Input: part model. Units: mm. Frame: model coordinates. Give positions to 0.01 mm unless a question says otherwise; leave off trailing zeros. Loops run counter-clockwise (first coordinate to the right, second up) from the corner with the lowest first, then second, coordinate; pieces in that order, holes last. Notation, with made-up numbers: (22, -37) -> (35, -37) arc R11 cw to (35, -19) -> close; hole circle Ø5 at (-17.5, 66). An arc over 180 degrees is marked (long way). Use CSV: the item, a comma, the result in double quotes.
```python
from build123d import *

# Parameters (mm, degrees)
SKETCH_1_R                       = 40.5
SKETCH_1_R_2                     = 34
SKETCH_1_R_3                     = 1.5
EXTRUDE_1_DEPTH                  = 2
CUT_EXTRUDE_1_DEPTH              = 58.310557492
FILLET_1_R                       = 1
PATTERN_CIRCULAR_1_COUNT         = 11
FILLET_1_OF_PATTERN_CIRCULAR_1_R = 1


with BuildPart() as part:
    # Sketch 1 → Extrude 1 (new body)
    with BuildSketch(Plane.XY):
        Circle(SKETCH_1_R)
        Circle(SKETCH_1_R_2, mode=Mode.SUBTRACT)
        with Locations((0, -38)):
            Circle(SKETCH_1_R_3, mode=Mode.SUBTRACT)
        with Locations((-20.544351063, -31.967634248)):
            Circle(SKETCH_1_R_3, mode=Mode.SUBTRACT)
        with Locations((-34.566015823, -15.785770494)):
            Circle(SKETCH_1_R_3, mode=Mode.SUBTRACT)
        with Locations((-37.613214791, 5.407963854)):
            Circle(SKETCH_1_R_3, mode=Mode.SUBTRACT)
        with Locations((-28.718483825, 24.88470789)):
            Circle(SKETCH_1_R_3, mode=Mode.SUBTRACT)
        with Locations((-10.70583716, 36.460732997)):
            Circle(SKETCH_1_R_3, mode=Mode.SUBTRACT)
        with Locations((10.70583716, 36.460732997)):
            Circle(SKETCH_1_R_3, mode=Mode.SUBTRACT)
        with Locations((28.718483825, 24.88470789)):
            Circle(SKETCH_1_R_3, mode=Mode.SUBTRACT)
        with Locations((37.613214791, 5.407963854)):
            Circle(SKETCH_1_R_3, mode=Mode.SUBTRACT)
        with Locations((34.566015823, -15.785770494)):
            Circle(SKETCH_1_R_3, mode=Mode.SUBTRACT)
        with Locations((20.544351063, -31.967634248)):
            Circle(SKETCH_1_R_3, mode=Mode.SUBTRACT)
    extrude(amount=EXTRUDE_1_DEPTH)

    # Sketch 2 → Cut-Extrude 1 (cut, through all)
    with BuildSketch(Plane.XY.offset(2)):
        with BuildLine():
            Line((-7.875033409, 38.707025833), (-6.977877705, 34.297364662))
            ThreePointArc((-6.977877705, 34.297364662), (0, 35), (6.977877705, 34.297364662))
            Line((6.977877705, 34.297364662), (7.875033409, 38.707025833))
            ThreePointArc((7.875033409, 38.707025833), (0, 39.5), (-7.875033409, 38.707025833))
        make_face()
    cut_extrude_1 = extrude(amount=-CUT_EXTRUDE_1_DEPTH, mode=Mode.SUBTRACT)

    # Fillet 1
    fillet_1_edges = [part.edges().sort_by_distance(p)[0] for p in [
        (-7.875033409, 38.707025833, 1),
        (7.875033409, 38.707025833, 1),
        (6.977877705, 34.297364662, 1),
        (-6.977877705, 34.297364662, 1),
    ]]
    fillet(fillet_1_edges, radius=FILLET_1_R)

    # Pattern Circular 1: Cut-Extrude 1 ×11 about axis
    pattern_circular_1_axis = Axis((0, 0, 0), (0, 0, 1))
    for i in range(1, PATTERN_CIRCULAR_1_COUNT):
        add(cut_extrude_1.rotate(pattern_circular_1_axis, i * 360 / PATTERN_CIRCULAR_1_COUNT), mode=Mode.SUBTRACT)

    # Fillet 1 of Pattern Circular 1
    fillet_1_of_pattern_circular_1_edges = [part.edges().sort_by_distance(p)[0] for p in [
        (-27.551497764, 28.304857727, 1),
        (-14.30169841, 36.819986727, 1),
        (-12.672390997, 32.625304695, 1),
        (-24.412719538, 25.080253682, 1),
        (-38.480556248, 8.916097286, 1),
        (-31.937742036, 23.242861993, 1),
        (-28.299265095, 20.594941007, 1),
        (-34.09669541, 7.900339367, 1),
        (-37.192310014, -13.303461046, 1),
        (-39.433778227, 2.286292803, 1),
        (-34.941322479, 2.025829066, 1),
        (-32.955211405, -11.787876876, 1),
        (-24.095768139, -31.299264493, 1),
        (-34.409868456, -19.396158198, 1),
        (-30.48975686, -17.18646929, 1),
        (-21.35068063, -27.7335255, 1),
        (-3.348990132, -39.357772613, 1),
        (-18.461068579, -34.920466018, 1),
        (-16.357908867, -30.942185079, 1),
        (-2.967459611, -34.873975733, 1),
        (18.461068579, -34.920466018, 1),
        (3.348990132, -39.357772613, 1),
        (2.967459611, -34.873975733, 1),
        (16.357908867, -30.942185079, 1),
        (34.409868456, -19.396158198, 1),
        (24.095768139, -31.299264493, 1),
        (21.35068063, -27.7335255, 1),
        (30.48975686, -17.18646929, 1),
        (39.433778227, 2.286292803, 1),
        (37.192310014, -13.303461046, 1),
        (32.955211405, -11.787876876, 1),
        (34.941322479, 2.025829066, 1),
        (31.937742036, 23.242861993, 1),
        (38.480556248, 8.916097286, 1),
        (34.09669541, 7.900339367, 1),
        (28.299265095, 20.594941007, 1),
        (14.30169841, 36.819986727, 1),
        (27.551497764, 28.304857727, 1),
        (24.412719538, 25.080253682, 1),
        (12.672390997, 32.625304695, 1),
    ]]
    fillet(fillet_1_of_pattern_circular_1_edges, radius=FILLET_1_OF_PATTERN_CIRCULAR_1_R)


solid = part.part
```
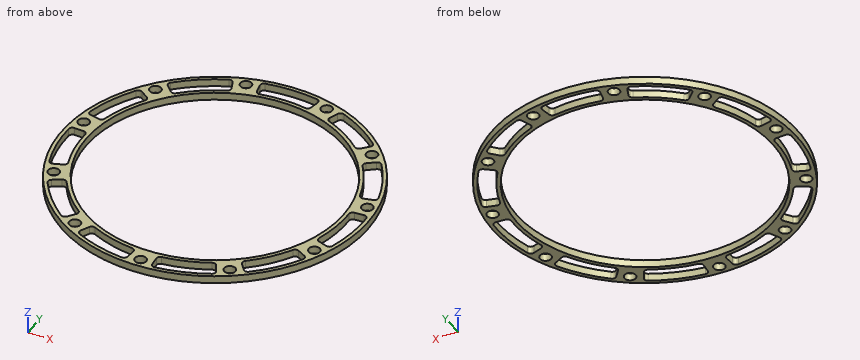
1) Ray query, line 1 (X direction, y = 1, z = 0.15); line 2 (X direction, y = 20, z = 1.25); line 3 (Y direction, x = 15.5, z = 0.5). Return the intervals inside material, ascending.
From the geometry:
line 1,"x = -40.49 to -39.49, -34.99 to -33.99, 33.99 to 34.99, 39.49 to 40.49"
line 2,"x = -35.22 to -34.06, -28.75 to -27.5, 27.5 to 28.75, 34.06 to 35.22"
line 3,"y = -37.42 to -36.33, -31.38 to -30.26, 30.26 to 31.38, 36.33 to 37.42"
2) Section query C-C (z = 0.3). Give the number of separate pieces and of enclosed holes in the cut face, then the cut area to 3 significant figures.
From the geometry:
separate pieces,"1"
enclosed holes,"23"
area,"713 mm^2"
3) Section query A-A (y = 0). Return loops of the section in (x, z).
From the geometry:
outline,"(-40.5, 0) -> (-39.5, 0) -> (-39.5, 2) -> (-40.5, 2) -> close; (-35, 0) -> (-34, 0) -> (-34, 2) -> (-35, 2) -> close; (34, 0) -> (35, 0) -> (35, 2) -> (34, 2) -> close; (39.5, 0) -> (40.5, 0) -> (40.5, 2) -> (39.5, 2) -> close"
4) Contact query for flat-ended pins moving along their axis: pin 1 (2.5 mm diameter, centred on x = 0, y = -38, fed in from +Z); pin 2 (1 mm diameter, centred on x = -26, z = 0.5, fed in from +Y). Output: stop coordinate, or through.
From the geometry:
pin 1,"passes through"
pin 2,"stops at y = 31.46"
5) Section query B-B (x = 0). Return loops of the section in (y, z).
From the geometry:
outline,"(-40.5, 0) -> (-39.5, 0) -> (-39.5, 2) -> (-40.5, 2) -> close; (-36.5, 0) -> (-34, 0) -> (-34, 2) -> (-36.5, 2) -> close; (34, 0) -> (35, 0) -> (35, 2) -> (34, 2) -> close; (39.5, 0) -> (40.5, 0) -> (40.5, 2) -> (39.5, 2) -> close"
